```python
from build123d import *

# Parameters (mm, degrees)
SKETCH1_W           = 10.3
SKETCH1_H           = 4
BOSS_EXTRUDE1_DEPTH = 3.7
CUT_EXTRUDE2_DEPTH  = 94.801132722
CUT_EXTRUDE3_DEPTH  = 94.801132722
CUT_EXTRUDE4_DEPTH  = 94.801132722


with BuildPart() as part:
    # Sketch1 → Boss-Extrude1 (new body)
    with BuildSketch(Plane.XY):
        Polygon((63, -54.75), (24.86, -54.75), (24.86, -65.95), (8.26, -65.95), (8.26, -54.75), (-8.26, -54.75), (-8.26, -65.95), (-24.86, -65.95), (-24.86, -54.75), (-63, -54.75), (-63, -32.25), (-66.6, -32.25), (-66.6, -16.65), (-63, -16.65), (-63, 16.65), (-66.6, 16.65), (-66.6, 32.25), (-63, 32.25), (-63, 54.75), (-24.86, 54.75), (-24.86, 65.95), (-8.26, 65.95), (-8.26, 54.75), (8.26, 54.75), (8.26, 65.95), (24.86, 65.95), (24.86, 54.75), (63, 54.75), (63, 32.25), (66.6, 32.25), (66.6, 16.65), (63, 16.65), (63, -16.65), (66.6, -16.65), (66.6, -32.25), (63, -32.25), align=None)
        with Locations((-17.042316358, 60.75)):
            Rectangle(SKETCH1_W, SKETCH1_H, mode=Mode.SUBTRACT)
        with Locations((17.042316358, 60.75)):
            Rectangle(SKETCH1_W, SKETCH1_H, mode=Mode.SUBTRACT)
        with Locations((17.042316358, -60.75)):
            Rectangle(SKETCH1_W, SKETCH1_H, mode=Mode.SUBTRACT)
        with Locations((-17.042316358, -60.75)):
            Rectangle(SKETCH1_W, SKETCH1_H, mode=Mode.SUBTRACT)
    extrude(amount=BOSS_EXTRUDE1_DEPTH)

    # Sketch2 → Cut-Extrude2 (cut, through all)
    with BuildSketch(Plane.XY.offset(3.7)):
        with BuildLine():
            Line((52.1, 45.75), (-52.1, 45.75))
            ThreePointArc((-52.1, 45.75), (-53.6, 47.25), (-52.1, 48.75))
            Line((-52.1, 48.75), (52.1, 48.75))
            ThreePointArc((52.1, 48.75), (53.6, 47.25), (52.1, 45.75))
        make_face()
    extrude(amount=-CUT_EXTRUDE2_DEPTH, mode=Mode.SUBTRACT)

    # Sketch2<3> → Cut-Extrude3 (cut, through all)
    with BuildSketch(Plane.XY.offset(3.7)):
        with BuildLine():
            Line((52.1, 45.75), (-52.1, 45.75))
            ThreePointArc((-52.1, 45.75), (-53.6, 47.25), (-52.1, 48.75))
            Line((-52.1, 48.75), (52.1, 48.75))
            ThreePointArc((52.1, 48.75), (53.6, 47.25), (52.1, 45.75))
        make_face()
        with BuildLine():
            Line((52.1, 40.75), (-52.1, 40.75))
            ThreePointArc((-52.1, 40.75), (-53.6, 42.25), (-52.1, 43.75))
            Line((-52.1, 43.75), (52.1, 43.75))
            ThreePointArc((52.1, 43.75), (53.6, 42.25), (52.1, 40.75))
        make_face()
        with BuildLine():
            Line((52.1, 35.75), (-52.1, 35.75))
            ThreePointArc((-52.1, 35.75), (-53.6, 37.25), (-52.1, 38.75))
            Line((-52.1, 38.75), (52.1, 38.75))
            ThreePointArc((52.1, 38.75), (53.6, 37.25), (52.1, 35.75))
        make_face()
        with BuildLine():
            Line((52.1, 30.75), (-52.1, 30.75))
            ThreePointArc((-52.1, 30.75), (-53.6, 32.25), (-52.1, 33.75))
            Line((-52.1, 33.75), (52.1, 33.75))
            ThreePointArc((52.1, 33.75), (53.6, 32.25), (52.1, 30.75))
        make_face()
        with BuildLine():
            Line((52.1, 25.75), (-52.1, 25.75))
            ThreePointArc((-52.1, 25.75), (-53.6, 27.25), (-52.1, 28.75))
            Line((-52.1, 28.75), (52.1, 28.75))
            ThreePointArc((52.1, 28.75), (53.6, 27.25), (52.1, 25.75))
        make_face()
        with BuildLine():
            Line((52.1, 20.75), (-52.1, 20.75))
            ThreePointArc((-52.1, 20.75), (-53.6, 22.25), (-52.1, 23.75))
            Line((-52.1, 23.75), (52.1, 23.75))
            ThreePointArc((52.1, 23.75), (53.6, 22.25), (52.1, 20.75))
        make_face()
        with BuildLine():
            Line((52.1, 15.75), (-52.1, 15.75))
            ThreePointArc((-52.1, 15.75), (-53.6, 17.25), (-52.1, 18.75))
            Line((-52.1, 18.75), (52.1, 18.75))
            ThreePointArc((52.1, 18.75), (53.6, 17.25), (52.1, 15.75))
        make_face()
        with BuildLine():
            Line((52.1, 10.75), (-52.1, 10.75))
            ThreePointArc((-52.1, 10.75), (-53.6, 12.25), (-52.1, 13.75))
            Line((-52.1, 13.75), (52.1, 13.75))
            ThreePointArc((52.1, 13.75), (53.6, 12.25), (52.1, 10.75))
        make_face()
        with BuildLine():
            Line((-25.5, -44.45), (-25.5, -0.75))
            ThreePointArc((-25.5, -0.75), (-24.2, 0.55), (-22.9, -0.75))
            Line((-22.9, -0.75), (-22.9, -44.45))
            ThreePointArc((-22.9, -44.45), (-24.2, -45.75), (-25.5, -44.45))
        make_face()
        with BuildLine():
            Line((-20, -44.45), (-20, -0.75))
            ThreePointArc((-20, -0.75), (-18.7, 0.55), (-17.4, -0.75))
            Line((-17.4, -0.75), (-17.4, -44.45))
            ThreePointArc((-17.4, -44.45), (-18.7, -45.75), (-20, -44.45))
        make_face()
        with BuildLine():
            Line((-14.5, -44.45), (-14.5, -0.75))
            ThreePointArc((-14.5, -0.75), (-13.2, 0.55), (-11.9, -0.75))
            Line((-11.9, -0.75), (-11.9, -44.45))
            ThreePointArc((-11.9, -44.45), (-13.2, -45.75), (-14.5, -44.45))
        make_face()
        with BuildLine():
            Line((-9, -44.45), (-9, -0.75))
            ThreePointArc((-9, -0.75), (-7.7, 0.55), (-6.4, -0.75))
            Line((-6.4, -0.75), (-6.4, -44.45))
            ThreePointArc((-6.4, -44.45), (-7.7, -45.75), (-9, -44.45))
        make_face()
        with BuildLine():
            Line((-3.5, -44.45), (-3.5, -0.75))
            ThreePointArc((-3.5, -0.75), (-2.2, 0.55), (-0.9, -0.75))
            Line((-0.9, -0.75), (-0.9, -44.45))
            ThreePointArc((-0.9, -44.45), (-2.2, -45.75), (-3.5, -44.45))
        make_face()
        with BuildLine():
            Line((2, -44.45), (2, -0.75))
            ThreePointArc((2, -0.75), (3.3, 0.55), (4.6, -0.75))
            Line((4.6, -0.75), (4.6, -44.45))
            ThreePointArc((4.6, -44.45), (3.3, -45.75), (2, -44.45))
        make_face()
        with BuildLine():
            Line((7.5, -44.45), (7.5, -0.75))
            ThreePointArc((7.5, -0.75), (8.8, 0.55), (10.1, -0.75))
            Line((10.1, -0.75), (10.1, -44.45))
            ThreePointArc((10.1, -44.45), (8.8, -45.75), (7.5, -44.45))
        make_face()
        with BuildLine():
            Line((13, -44.45), (13, -0.75))
            ThreePointArc((13, -0.75), (14.3, 0.55), (15.6, -0.75))
            Line((15.6, -0.75), (15.6, -44.45))
            ThreePointArc((15.6, -44.45), (14.3, -45.75), (13, -44.45))
        make_face()
        with BuildLine():
            Line((18.5, -44.45), (18.5, -0.75))
            ThreePointArc((18.5, -0.75), (19.8, 0.55), (21.1, -0.75))
            Line((21.1, -0.75), (21.1, -44.45))
            ThreePointArc((21.1, -44.45), (19.8, -45.75), (18.5, -44.45))
        make_face()
    extrude(amount=-CUT_EXTRUDE3_DEPTH, mode=Mode.SUBTRACT)

    # Sketch4 → Cut-Extrude4 (cut, through all)
    with BuildSketch(Plane.XY.offset(3.7)):
        Polygon((-55.935998942, 8.25), (-55.935998942, -50.75), (-49.192042483, -50.75), (-49.192042483, -46.05), (-40.435998942, -46.05), (-40.435998942, -32.45), (-46.435998942, -32.45), (-46.435998942, -10.05), (-40.435998942, -10.05), (-40.435998942, 3.55), (-46.435998942, 3.55), (-46.435998942, 8.25), align=None)
        Polygon((46.435998942, 3.55), (46.435998942, 8.25), (55.935998942, 8.25), (55.935998942, -50.75), (49.192042483, -50.75), (49.192042483, -46.05), (40.435998942, -46.05), (40.435998942, -32.45), (46.435998942, -32.45), (46.435998942, -10.05), (40.435998942, -10.05), (40.435998942, 3.55), align=None)
    extrude(amount=-CUT_EXTRUDE4_DEPTH, mode=Mode.SUBTRACT)


solid = part.part
```
Here's how the part is built. I have some questions about the finished solid (model axes, mm). A direction names the side the tool comes from. Round coordinates to 2 decimals unless told otherwise and drop trailing zeros. Order: outer loops, then holes, each group sorted by start corner. A loop starts at its lowest first (then second) coordinate and runs counter-clockwise, first axis right, second up. Notation, with made-up numbers: M -8.5,65 L 4.5,65 A17 ccw 4.5,82 Z; hole C 7,29.25 d2. An arc over 180 degrees is marked long. One line per question, with ' | ' between items.
1) I need wall thicknesses on line 1 along X through (y, z) = (3, 2.35); line 2 along X through (y, z) = (6, 1.6); line 3 along X through (y, z) = (58, 2.4). Which ranges of each line are inside material? Lowest first, please.
Working result:
line 1: -63 to -55.94, -40.44 to 40.44, 55.94 to 63 | line 2: -63 to -55.94, -46.44 to 46.44, 55.94 to 63 | line 3: -24.86 to -8.26, 8.26 to 24.86
2) If we mould it in two halves opening along X, with no side actions, what happens to faces 5 (the face through (40.436, -3, 2)), 6 (the face through (16, 65.95, 2)), 7 (the face through (40.436, -39, 2)), 8 (the face through (-63, -44, 2))? For each: +X half, -X half, draft (parallel to the pull), parting line (faces both ways), or undercut.
Working result:
face 5: undercut | face 6: draft | face 7: undercut | face 8: -X half
3) For pin 1 Ø1.1 at (x, z) = (44, 2.5) entering from +Y; pin 2 Ø2 at (y, z) = (6.5, 1) entering from -X, each with a flat end and sliding along its axis, tell me the tip position at first contact or that it passes through.
Working result:
pin 1: y = 54.75 | pin 2: x = -63
4) I want a section at A-A, the plane y = 12.25. Write out the boundary of the cut face in (x, z), then the cut area to 3 significant figures.
Working result:
outline: M -63,0 L -53.6,0 L -53.6,3.7 L -63,3.7 Z; M 53.6,0 L 63,0 L 63,3.7 L 53.6,3.7 Z | area: 69.6 mm²
5) I want a section at B-B, the plane z = 2. State how many separate pieces and enclosed holes the cut face has, then the cut area to 3 significant figures.
Working result:
separate pieces: 1 | enclosed holes: 23 | area: 9,550 mm²
6) For faces 1 (the face through (-63, 0, 2)), 2 (the face through (63, 44, 2)), 3 (the face through (-43, -10.05, 2)), 4 (the face through (-8.26, 60, 2)), which set-ups out of +Z, -Z, +X, -X, +Y, -Y let a thin tool reach every point of the face, with its end or its side?
Working result:
face 1: +Z, -Z, -X | face 2: +Z, -Z, +X, +Y | face 3: +Z, -Z | face 4: +Z, -Z, +Y
